Design review of the part built by this model. Coordinates are the model's own, in mm. Face numbers are marked on the shaded views. A direction names the side the tool comes from. Round coordinates to 2 decimals unless told otherwise and drop trailing zeros. Loops run counter-clockwise (first coordinate to the right, second up) from the corner with the lowest first, then second, coordinate; pieces in that order, holes last. Notation, with made-up numbers: (30, 39) - (49, 39) arc R22 ccw to (49, 73) - close; hole circle Ø8 at (50, 32). An arc over 180 degrees is marked (long way). Answer as CSV lines item,"result". Start each with the question number.
(1) Consider section B-B (z = -2.5). Give the boundary of the cut face in (x, y).
(2) Consider section C-C (x = -0.25). Give the boundary of the cut face in (y, z), and give its area (3 significant figures).
(3) Consider section A-A (x = -8). Give the boundary of the cut face in (y, z), and give its area (3 significant figures).
(4) For the marked faces 1, 2 and 3, list the 3-axis set-ups (+Z, -Z, +X, -X, +Y, -Y) from which the entire face can be reached by the end or side of a thin tool; tool diameter is ignored.
(5) Wall thickness on L1, parallel to Z at x = -7.25, y = 0; L2, parallel to X at y = -3, z = 3.5; L3, parallel to X at y = -0.75, z = -1: over which ranges is each line inside the solid? List them lowest first.
(6) Mouldability with a two-part tool opening along Y and no side actions: class the marked faces 4, 5 and 6 as released by +Y, released by -Y, zero draft, split by the parting line, or undercut.
(7) Consider section D-D (z = 4). Give the boundary of the cut face in (x, y).
(8) For P1, Ø1.5, axis at y = -1, z = -2.5, coming from the +X side; P2, Ø3, axis at x = -4, y = 3, coming from the +Z side; P3, Ø1, axis at x = -6.5, z = 1.5, coming from the -Y side, all flat-tipped, find the tip position at first contact; note any pin that passes through.
Autodesk Inventor part; units mm, degrees
ref_plane "YZ Plane" through (0, 0, 0) normal (1, 0, 0) x (0, 1, 0)
ref_plane "XZ Plane" through (0, 0, 0) normal (0, 1, 0) x (-1, 0, 0)
ref_plane "XY Plane" through (0, 0, 0) normal (0, 0, 1) x (1, 0, 0)
sketch "Sketch_1" plane through (0, 0, 0) normal (0, 0, 1) x (1, 0, 0)
  line L0 (4, 0) -> (-8.8, 0)
  line L1 (-8.8, 0) -> (-8.8, 5)
  line L2 (-8.8, 5) -> (-6, 5)
  line L3 (-6, 5) -> (-6, 3)
  line L4 (-6, 3) -> (0, 3)
  line L5 (0, 3) -> (0, 2)
  line L6 (0, 2) -> (3.5705, 2)
  line L7 (3.5705, 2) -> (4, 1.5705)
  line L8 (4, 1.5705) -> (4, 0)
  line L9 (4, 0) -> (-8.8, 0)
revolve "Revolution1" add sketch "Sketch_1" angle 360 about axis through (4, 0, 0) along (1, 0, 0)
thread "Thread1"
sketch "Sketch_2" plane through (-8.8, 0, 0) normal (-1, 0, 0) x (0, 1, 0)
  line L0 (-1.4434, 0) -> (-0.7217, -1.25)
  line L1 (-0.7217, -1.25) -> (0.7217, -1.25)
  line L2 (0.7217, -1.25) -> (1.4434, 0)
  line L3 (1.4434, 0) -> (0.7217, 1.25)
  line L4 (0.7217, 1.25) -> (-0.7217, 1.25)
  line L5 (-0.7217, 1.25) -> (-1.4434, 0)
extrude "Extrusion1" cut sketch "Sketch_2" against normal blind 2.5
sketch "Sketch_3" plane through (0, 0, 0) normal (0, 0, 1) x (1, 0, 0)
  line L0 (-5.5783, 0) -> (-6.3, 0)
  line L1 (-6.3, 0) -> (-6.3, 1.25)
  line L2 (-6.3, 1.25) -> (-5.5783, 0)
  line L3 (-5.5783, 0) -> (-6.3, 0)
revolve "Revolution2" cut sketch "Sketch_3" angle 360 about axis through (-5.5783, 0, 0) along (1, 0, 0)
properties part number "DBS4-6-4"
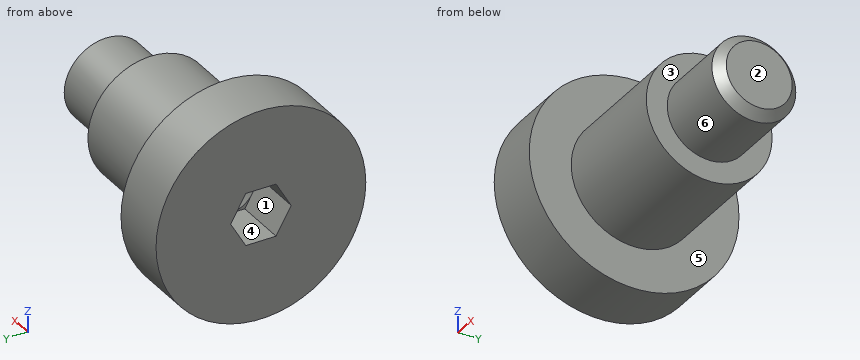
Determined:
1,outline,"(-8.8, -4.33) - (-6, -4.33) - (-6, -1.66) - (0, -1.66) - (0, 1.66) - (-6, 1.66) - (-6, 4.33) - (-8.8, 4.33) - close"
2,outline,"circle Ø6 at (0, 0)"
2,area,"28.3 mm^2"
3,outline,"circle Ø10 at (0, 0); hole (-1.44, 0) - (-0.72, -1.25) - (0.72, -1.25) - (1.44, 0) - (0.72, 1.25) - (-0.72, 1.25) - close"
3,area,"73.1 mm^2"
4,face 1,"-X"
4,face 2,"+Z, -Z, +X, +Y, -Y"
4,face 3,"+X"
5,L1,"z = -5 to -1.25, 1.25 to 5"
5,L2,"x = -8.8 to -6"
5,L3,"x = -6.3 to 4"
6,face 4,"undercut"
6,face 5,"zero draft"
6,face 6,"split by the parting line"
7,outline,"(-8.8, -3) - (-6, -3) - (-6, 3) - (-8.8, 3) - close"
8,P1,"stops at x = 3.63"
8,P2,"stops at z = 2.6"
8,P3,"stops at y = -4.9"
